Design review of the part shown in the three views and the two pictorial views. Dimensions are in mm from the part's minimum x, y and z. A direction names the side the tool comes from. Coordinates: 2 decimals unless noted, no trailing zeros. Loops run counter-clockwise (first coordinate to the right, second up) from the corner with the lowest first, then second, coordinate; pieces in that order, holes last.
Q1. Add section D-D on y = 6. Give the boundary of the cut face in (x, z), and give its area (3 significant figures).
Q2. Add section A-A on y = 15. Give the boundary of the cut face in (x, z).
Q3. For P1, Ø6, axis at x = 87.5, z = 34.5, coming from the -Y side; P2, Ø11.5, axis at x = 44.5, y = 21.5, coming from the -Z side; P3, Ø4, axis at y = 9.5, z = 36.5, coming from the -X side, all flat-tipped, find the tip position at first contact; note any pin that passes through.
Q4. Add section B-B on x = 85. Give the boundary of the cut face in (y, z), and give its area (3 significant figures).
Q5. Wall thickness on probe 1 along X at (y, z) = (28, 11); probe 2 along Z at (x, y) = (44, 31.5); probe 3 along Y at (x, z) = (5.5, 32): over which ranges is each line inside the solid? List them lowest first.
Q6. Machinability: for the marked faces 1, 2, 3, 4 and 5, which of the approach directions +Z, -Z, +X, -X, +Y, -Y give a long, thin tool a straight path to every point of the face, cutting with its end or side? Answer none if there is none.
Q7. Add section C-C on z = 32.5. Give the boundary of the cut face in (x, y).
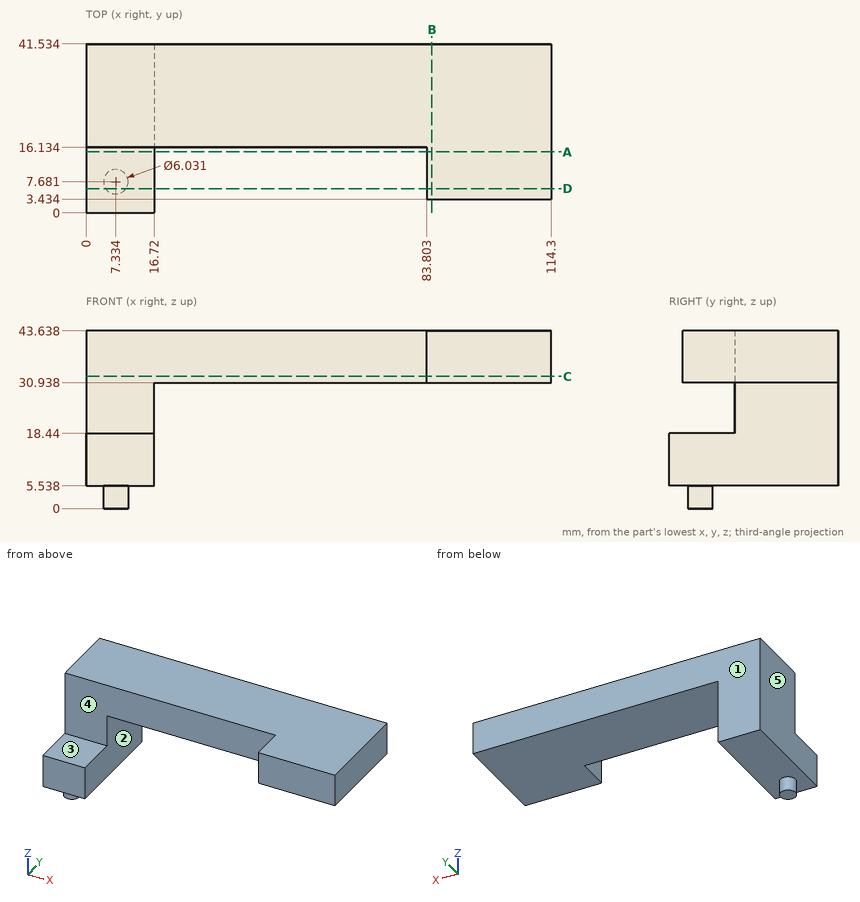
Entries:
1. outline: (0, 5.54) - (4.83, 5.54) - (4.83, 0) - (9.84, 0) - (9.84, 5.54) - (16.72, 5.54) - (16.72, 18.44) - (0, 18.44) - close; (83.8, 30.94) - (114.3, 30.94) - (114.3, 43.64) - (83.8, 43.64) - close
1. area: 631 mm2
2. outline: (0, 5.54) - (16.72, 5.54) - (16.72, 18.44) - (0, 18.44) - close; (83.8, 30.94) - (114.3, 30.94) - (114.3, 43.64) - (83.8, 43.64) - close
3. P1: stops at y = 3.43
3. P2: stops at z = 30.94
3. P3: stops at x = 83.8
4. outline: (3.43, 30.94) - (41.53, 30.94) - (41.53, 43.64) - (3.43, 43.64) - close
4. area: 484 mm2
5. probe 1: x = 0 to 16.72
5. probe 2: z = 30.94 to 43.64
5. probe 3: y = 16.13 to 41.53
6. face 1: +Z, -Z, +X, -X, +Y
6. face 2: -Z, +X, +Y, -Y
6. face 3: +Z, +X, -X, -Y
6. face 4: +Z, -X, -Y
6. face 5: +Z, -Z, -X, +Y, -Y
7. outline: (0, 16.13) - (83.8, 16.13) - (83.8, 3.43) - (114.3, 3.43) - (114.3, 41.53) - (0, 41.53) - close
